from build123d import *

# Parameters (mm, degrees)
SKETCH1_R           = 25
BOSS_EXTRUDE1_DEPTH = 2
SKETCH2_R           = 1.05
CUT_EXTRUDE1_DEPTH  = 3
SKETCH3_R           = 4
CUT_EXTRUDE2_DEPTH  = 1
SKETCH4_R           = 3
SKETCH4_R_2         = 1.95
BOSS_EXTRUDE2_DEPTH = 6
FILLET1_R           = 1
SKETCH5_R           = 2.05
CUT_EXTRUDE3_DEPTH  = 9
SKETCH7_R           = 1.55
CUT_EXTRUDE4_DEPTH  = 9


with BuildPart() as part:
    # Sketch1 → Boss-Extrude1 (new body)
    with BuildSketch(Plane(origin=(0, 0, 0), x_dir=(1, 0, 0), z_dir=(0, 1, 0))):
        Circle(SKETCH1_R)
    extrude(amount=BOSS_EXTRUDE1_DEPTH)

    # Sketch2 → Cut-Extrude1 (cut, through all)
    with BuildSketch(Plane(origin=(0, 2, 0), x_dir=(1, 0, 0), z_dir=(0, 1, 0))):
        with Locations((-2.066368974, 7.209723938)):
            Circle(SKETCH2_R)
        with Locations((7.209723938, 2.066368974)):
            Circle(SKETCH2_R)
        with Locations((2.066368974, -7.209723938)):
            Circle(SKETCH2_R)
        with Locations((-7.209723938, -2.066368974)):
            Circle(SKETCH2_R)
    extrude(amount=-CUT_EXTRUDE1_DEPTH, mode=Mode.SUBTRACT)

    # Sketch3 → Cut-Extrude2 (cut)
    with BuildSketch(Plane(origin=(0, 2, 0), x_dir=(1, 0, 0), z_dir=(0, 1, 0))):
        Circle(SKETCH3_R)
        with Locations((17.056217149, -3.916051143)):
            Circle(SKETCH3_R)
        with Locations((9.291500489, -14.829633126)):
            Circle(SKETCH3_R)
        with Locations((-3.916051143, -17.056217149)):
            Circle(SKETCH3_R)
        with Locations((-14.829633126, -9.291500489)):
            Circle(SKETCH3_R)
        with Locations((-17.056217149, 3.916051143)):
            Circle(SKETCH3_R)
        with Locations((-9.291500489, 14.829633126)):
            Circle(SKETCH3_R)
        with Locations((3.916051143, 17.056217149)):
            Circle(SKETCH3_R)
        with Locations((14.829633126, 9.291500489)):
            Circle(SKETCH3_R)
    extrude(amount=-CUT_EXTRUDE2_DEPTH, mode=Mode.SUBTRACT)

    # Sketch4 → Boss-Extrude2 (add)
    with BuildSketch(Plane.XZ):
        with Locations((2.066368974, 7.209723938)):
            Circle(SKETCH4_R)
        with Locations((2.066368974, 7.209723938)):
            Circle(SKETCH4_R_2, mode=Mode.SUBTRACT)
        with Locations((7.209723938, -2.066368974)):
            Circle(SKETCH4_R)
        with Locations((7.209723938, -2.066368974)):
            Circle(SKETCH4_R_2, mode=Mode.SUBTRACT)
        with Locations((-2.066368974, -7.209723938)):
            Circle(SKETCH4_R)
        with Locations((-2.066368974, -7.209723938)):
            Circle(SKETCH4_R_2, mode=Mode.SUBTRACT)
        with Locations((-7.209723938, 2.066368974)):
            Circle(SKETCH4_R)
        with Locations((-7.209723938, 2.066368974)):
            Circle(SKETCH4_R_2, mode=Mode.SUBTRACT)
    extrude(amount=BOSS_EXTRUDE2_DEPTH)

    # Fillet1
    fillet1_edges = [part.edges().sort_by_distance(p)[0] for p in [
        (-0.933631026, 0, 7.209723938),
        (4.209723938, 0, -2.066368974),
        (-5.066368974, 0, -7.209723938),
        (-10.209723938, 0, 2.066368974),
    ]]
    fillet(fillet1_edges, radius=FILLET1_R)

    # Sketch5 → Cut-Extrude3 (cut, through all)
    with BuildSketch(Plane(origin=(0, 2, 0), x_dir=(1, 0, 0), z_dir=(0, 1, 0))):
        with Locations((-11.594389967, -16.296322324)):
            Circle(SKETCH5_R)
        with Locations((-19.721711793, -3.324768254)):
            Circle(SKETCH5_R)
        with Locations((-16.296322324, 11.594389967)):
            Circle(SKETCH5_R)
        with Locations((-3.324768254, 19.721711793)):
            Circle(SKETCH5_R)
        with Locations((11.594389967, 16.296322324)):
            Circle(SKETCH5_R)
        with Locations((19.721711793, 3.324768254)):
            Circle(SKETCH5_R)
        with Locations((16.296322324, -11.594389967)):
            Circle(SKETCH5_R)
        with Locations((3.324768254, -19.721711793)):
            Circle(SKETCH5_R)
    extrude(amount=-CUT_EXTRUDE3_DEPTH, mode=Mode.SUBTRACT)

    # Sketch7 → Cut-Extrude4 (cut, through all)
    with BuildSketch(Plane(origin=(0, 2, -2), x_dir=(1, 0, 0), z_dir=(0, -1, 0))):
        with Locations((-3.636901173, 8.559188201)):
            Circle(SKETCH7_R)
        with Locations((6.559188201, 5.636901173)):
            Circle(SKETCH7_R)
        with Locations((3.636901173, -4.559188201)):
            Circle(SKETCH7_R)
        with Locations((-6.559188201, -1.636901173)):
            Circle(SKETCH7_R)
    extrude(amount=CUT_EXTRUDE4_DEPTH, mode=Mode.SUBTRACT)


solid = part.part
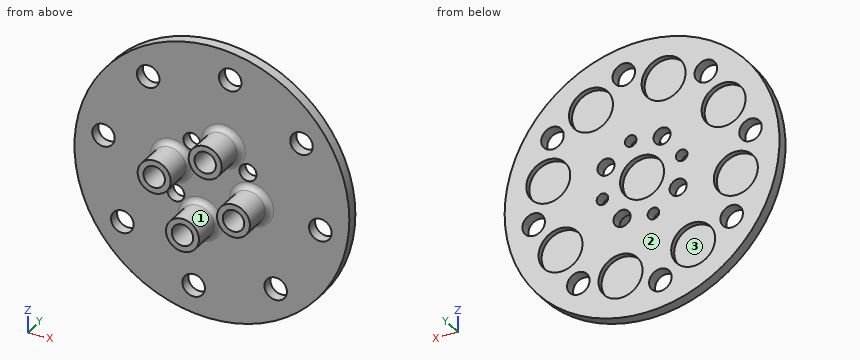
The listing builds one solid part. Answer for the finished solid, in the listing's coordinates (mm). Face numbers are marked on the shaded views. A direction names the side the tool comes from. Give positions to 0.01 mm unless a question says otherwise; leave off trailing zeros. Order: outer loops, then holes, each group sorted by start corner. A loop starts at its lowest first (then second) coordinate and runs counter-clockwise, first axis right, second up. Notation, with made-up numbers: (36, 18.5) - (62, 18.5) arc R6 cw to (62, 26.5) - close; hole circle Ø8 at (-27.5, -22.75). An arc over 180 degrees is marked (long way). One line per item, written item: value. Start each with the question number.
1) Given pin 1 Ø1 at (y, z) = (1, -10.5) entering from +X; pin 2 Ø3 at (x, z) = (-7.21, 2.07) entering from -Y; pin 3 Ø6.5 at (x, z) = (9.29, 14.83) entering from +Y; pin 4 Ø4 at (x, z) = (-3.64, 6.56) entering from +Y, each flat-ended and moving along its own axis, determine where each tip first touches the part or whether it passes through.
2) A cutting plane is placed at B-B on x = 7. State how many separate pieces and enclosed holes the cut face has, then the cut area to 3 significant figures.
3) A cutting plane is placed at A-A on y = -3.75. Give the vertices of the cut face in (x, z), then the cut area to 3 significant figures.
4) A tool of negligible diameter and unlimited length cuts with its end or side. For the marked faces 1, 2 and 3, from which of +Z, -Z, +X, -X, +Y, -Y can it reach the whole face along a straight path? Write none if from no direction.
5) Find the intervals of material crossed by L1, parallel to X at y = -2.5, z = 2; L2, parallel to X at y = 1.75, z = -18.5; L3, parallel to Z at x = -18, y = 1.5, in increasing order.
Answer sheet:
1. pin 1: stops at x = 22.91
1. pin 2: stops at y = 0
1. pin 3: stops at y = 1
1. pin 4: stops at y = 2
2. separate pieces: 3
2. enclosed holes: 0
2. area: 87.4 mm2
3. outline: circle Ø6 at (-7.21, 2.07); circle Ø6 at (-2.07, -7.21); circle Ø6 at (2.07, 7.21); circle Ø6 at (7.21, -2.07); hole circle Ø3.9 at (-7.21, 2.07); hole circle Ø3.9 at (-2.07, -7.21); hole circle Ø3.9 at (2.07, 7.21); hole circle Ø3.9 at (7.21, -2.07)
3. area: 65.3 mm2
4. face 1: -Y
4. face 2: +Z, -Z, +X, -X, +Y
4. face 3: +Y
5. L1: x = -10.21 to -9.16, -5.26 to -4.21
5. L2: x = -16.82 to -10.88, -7.7 to -4.97, -1.68 to 0.19, 7.65 to 16.82
5. L3: z = -17.35 to -12.73, -10.45 to -7.8, -0.03 to 2.21, 4.44 to 6.85, 11.73 to 17.35
